from build123d import *

# Parameters (mm, degrees)
BASEHEAD_DEPTH  = 15.3416
THDSCHPAT_COUNT = 19
THDSCHPAT_PITCH = 2.673684211


with BuildPart() as part:
    # Sketch1 → BaseHead (new body)
    with BuildSketch(Plane(origin=(0, 0, 0), x_dir=(0, 0, -1), z_dir=(1, 0, 0))):
        Polygon((16.6624, 9.620041125), (16.6624, -9.620041125), (0, -19.240082251), (-16.6624, -9.620041125), (-16.6624, 9.620041125), (0, 19.240082251), align=None)
    extrude(amount=BASEHEAD_DEPTH)

    # BodySke → BaseBody (revolve)
    with BuildSketch(Plane.XY):
        Polygon((0, 0), (116.9416, 0), (116.9416, 9.43229), (115.26139, 11.1125), (0, 11.1125), align=None)
    revolve(axis=Axis((0, 0, 0), (1, 0, 0)))

    # Sketch3 → HeadChamfer (revolve, cut)
    with BuildSketch(Plane.XY):
        Polygon((0, 16.6624), (5.154399751, 25.590082251), (5.154399751, 31.940082251), (-12.7, 31.940082251), (-12.7, 16.6624), align=None)
    revolve(axis=Axis((0, 0, 0), (1, 0, 0)), mode=Mode.SUBTRACT)

    # ThdSchSke → ThreadSchematic (revolve, cut)
    with BuildSketch(Plane.XY):
        Polygon((66.1416, -9.43229), (64.965104292, -11.1125), (64.965104292, -13.890625), (67.318095708, -13.890625), (67.318095708, -11.1125), align=None)
    threadschematic = revolve(axis=Axis((-3.175, 0, 0), (1, 0, 0)), mode=Mode.SUBTRACT)

    # ThdSchPat: ThreadSchematic ×19
    with Locations(*[(i * THDSCHPAT_PITCH, 0, 0) for i in range(1, THDSCHPAT_COUNT)]):
        add(threadschematic, mode=Mode.SUBTRACT)


solid = part.part
Work out the finished part from the listing and answer in its coordinate system (mm). A direction names the side the tool comes from. Coordinates: 2 decimals unless noted, no trailing zeros. Order: outer loops, then holes, each group sorted by start corner. A loop starts at its lowest first (then second) coordinate and runs counter-clockwise, first axis right, second up. Notation, with made-up numbers: (4, 89.25) - (56, 89.25) arc R34 ccw to (56, 123.25) - close; hole circle Ø2 at (61.5, 46.5). An arc over 180 degrees is marked (long way). Put each result on its own line as item: value. Start each with the question number.
1) Find the intervals of material crossed by line 1 (Y direction, x = 40, z = -0.5); line 2 (X direction, y = -8, z = -8); line 3 (Z direction, x = 109.5, y = -6), in increasing order. Write a range as from..to.
2) Find section B-B (x = 49). Give the vertices of the cut face in (y, z) (1 decimal), plus the area to 3 significant figures.
3) Find section A-A (x = 12.5). Give the vertices of the cut face in (y, z), plus the area to 3 significant figures.
4) For faces 1 (the flat face through (116.942, 0, 0)), 2 (the cylindrical face through (78.17, 10.6, 3.34)), determine the directions among +Z, -Z, +X, -X, +Y, -Y from which every point of the face is accessible in a straight line to the end or side of a thin tool.
5) Flat-ended cylindrical pins translate along their axes: pin 1 (1 mm diameter, centred on x = 90.5, z = -1, fed in from +Y); pin 2 (8 mm diameter, centred on x = 70, y = -12.5, fed in from -Z); pin 3 (2 mm diameter, centred on y = -13, z = 5, fed in from +X). Find the tip coordinate at first contact, or state that the pin passes through.
Results list:
1. line 1: y = -11.1..11.1
1. line 2: x = 0..15.34
1. line 3: z = -8.32..8.32
2. outline: circle Ø22.2 at (0, 0)
2. area: 388 mm^2
3. outline: (-19.24, 0) - (-9.62, -16.66) - (9.62, -16.66) - (19.24, 0) - (9.62, 16.66) - (-9.62, 16.66) - close
3. area: 962 mm^2
4. face 1: +Z, -Z, +X, +Y, -Y
4. face 2: +X
5. pin 1: stops at y = 10.52
5. pin 2: stops at z = -7.16
5. pin 3: stops at x = 15.34
